from build123d import *

# Parameters (mm, degrees)
SKETCH1_R           = 3.25
BOSS_EXTRUDE1_DEPTH = 3


with BuildPart() as part:
    # Sketch1 → Boss-Extrude1 (new body)
    with BuildSketch(Plane(origin=(0, 0, 0), x_dir=(1, 0, 0), z_dir=(0, 1, 0))):
        with BuildLine():
            Line((-180, 12.5), (180, 12.5))
            ThreePointArc((180, 12.5), (187.071067812, 9.571067812), (190, 2.5))
            Line((190, 2.5), (190, -2.5))
            ThreePointArc((190, -2.5), (187.071067812, -9.571067812), (180, -12.5))
            Line((180, -12.5), (-180, -12.5))
            ThreePointArc((-180, -12.5), (-187.071067812, -9.571067812), (-190, -2.5))
            Line((-190, -2.5), (-190, 2.5))
            ThreePointArc((-190, 2.5), (-187.071067812, 9.571067812), (-180, 12.5))
        make_face()
        with Locations((-180, 0)):
            Circle(SKETCH1_R, mode=Mode.SUBTRACT)
        with Locations((180, 0)):
            Circle(SKETCH1_R, mode=Mode.SUBTRACT)
    extrude(amount=BOSS_EXTRUDE1_DEPTH)


solid = part.part
Read the model definition and answer for the solid it produces. Units are mm, in the model's axes. Coordinates: 2 decimals unless noted, no trailing zeros. Order: outer loops, then holes, each group sorted by start corner. A loop starts at its lowest first (then second) coordinate and runs counter-clockwise, first axis right, second up. Notation, with made-up numbers: (-18, 19) - (35, 19) arc R25 ccw to (35, 51) - close; hole circle Ø5 at (-13, 76.25). An arc over 180 degrees is marked (long way). Use one line per item in the form item = value.
(1) Section A-A, the plane y = 2.25 is taken. Give the vertices of the cut face in (x, z).
Computed values:
outline = (-190, -2.5) arc R10 ccw to (-180, -12.5) - (180, -12.5) arc R10 ccw to (190, -2.5) - (190, 2.5) arc R10 ccw to (180, 12.5) - (-180, 12.5) arc R10 ccw to (-190, 2.5) - close; hole circle Ø6.5 at (-180, 0); hole circle Ø6.5 at (180, 0)
(2) Straight lines are drawn through the part: L1, parallel to X at y = 1.85, z = 0; L2, parallel to Z at x = -180, y = 2.2; L3, parallel to X at y = 1, z = 2. For each, find the intervals that lie inside material, in ascending order.
Computed values:
L1 = -190 to -183.25, -176.75 to 176.75, 183.25 to 190
L2 = -12.5 to -3.25, 3.25 to 12.5
L3 = -190 to -182.56, -177.44 to 177.44, 182.56 to 190
(3) For a pull along X with two mould halves and no side action, classify faces 1 (the face through (-176.9, 1.48, -0.98)), 2 (the face through (3, 3, 0)), 3 (the face through (187.15, 1.48, 9.49)) as pulls with the +X half, pulls with the -X half, needs draft (parallel to the pull), parting line crosses it, or undercut.
Computed values:
face_1 = undercut
face_2 = needs draft
face_3 = pulls with the +X half
